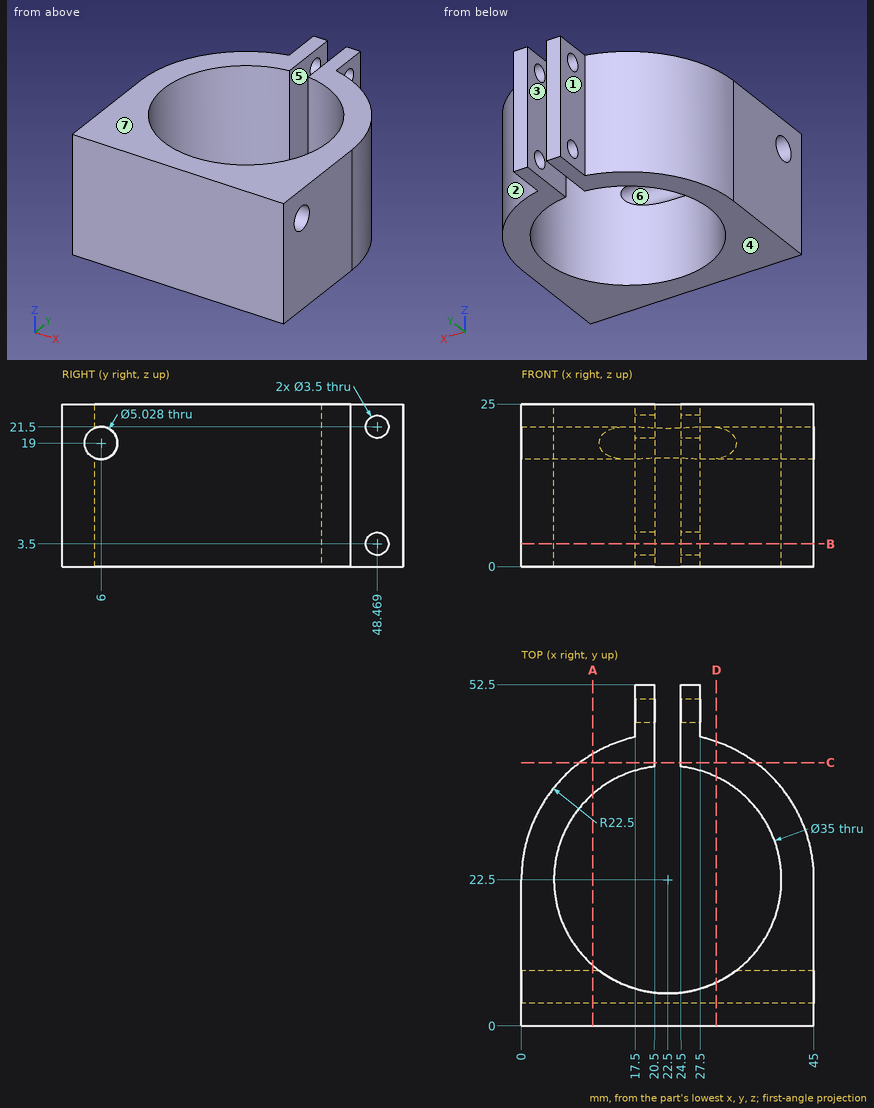
Design review of the part shown in the three views and the two pictorial views. Dimensions are in mm from the part's minimum x, y and z. A direction names the side the tool comes from. Coordinates: 2 decimals unless noted, no trailing zeros. Write each loop counter-clockwise with the first axis right and the second up, starting at its lowest first coordinate (ties: lowest second). Pieces come first, ordered by that corner, then holes.
(1) For pin 1 Ø3 at (y, z) = (48.47, 3.5) entering from -X; pin 2 Ø2 at (x, z) = (40.5, 16.5) entering from +Y; pin 3 Ø4 at (y, z) = (49, 7) entering from -X; pin 4 Ø10 at (y, z) = (36, 15) entering from -X, all flat-tipped, find the tip position at first contact; note any pin that passes through.
(2) Tool access review of the marked faces 1, 2 and 3: name each direction out of +Z, -Z, +X, -X, +Y, -Y from which nothing blocks a thin tool from reaching the whole face with its end or side.
(3) Add section B-B on z = 3.5. Give the boundary of the cut face in (x, y) (1 decimal), then the cut area to 3 significant figures.
(4) The part is to be moulded in two halves that separate along Z. For the marked faces 4, 5, 6 and 7, say which applies: +Z half, -Z half, draft (parallel to the pull), parting line (faces both ways), or undercut.
(5) Wall thickness on probe 1 along X at (y, z) = (22.5, 9); probe 2 along Z at (x, y) = (25.5, 47); probe 3 along X at (y, z) = (44.5, 8.25): over which ranges is each line inside the solid? List them lowest first.
(6) Add section D-D on x = 30. Give the boundary of the cut face in (y, z).
(7) Add section C-C on y = 40.5. Give the boundary of the cut face in (x, z), then the cut area to 3 significant figures.
(8) Add section A-A on x = 11. Give the boundary of the cut face in (y, z).
Answer sheet:
1. pin 1: passes through
1. pin 2: stops at y = 37.24
1. pin 3: stops at x = 17.5
1. pin 4: stops at x = 1.67
2. face 1: +Z, -Z, -X, +Y
2. face 2: +Z, -Z, +X, +Y
2. face 3: +Z, -Z, +Y
3. outline: (0, 0) - (45, 0) - (45, 22.5) arc R22.5 ccw to (27.5, 44.4) - (27.5, 46.7) - (24.5, 46.7) - (24.5, 39.9) arc R17.5 cw (long way) to (20.5, 39.9) - (20.5, 46.7) - (17.5, 46.7) - (17.5, 44.4) arc R22.5 ccw to (0, 22.5) - close; (17.5, 50.2) - (20.5, 50.2) - (20.5, 52.5) - (17.5, 52.5) - close; (24.5, 50.2) - (27.5, 50.2) - (27.5, 52.5) - (24.5, 52.5) - close
3. area: 851 mm2
4. face 4: -Z half
4. face 5: draft
4. face 6: undercut
4. face 7: +Z half
5. probe 1: x = 0 to 5, 40 to 45
5. probe 2: z = 0 to 2.55, 4.45 to 20.55, 22.45 to 25
5. probe 3: x = 17.5 to 20.5, 24.5 to 27.5
6. outline: (0, 0) - (6.69, 0) - (6.69, 16.58) arc R2.51 cw (long way) to (6.69, 21.42) - (6.69, 25) - (0, 25) - close; (38.31, 0) - (43.71, 0) - (43.71, 25) - (38.31, 25) - close
7. outline: (9, 0) - (20.5, 0) - (20.5, 25) - (9, 25) - close; (24.5, 0) - (36, 0) - (36, 25) - (24.5, 25) - close
7. area: 575 mm2
8. outline: (0, 0) - (9.31, 0) - (9.31, 25) - (0, 25) - close; (35.69, 0) - (41.84, 0) - (41.84, 25) - (35.69, 25) - close; hole circle Ø5.03 at (6, 19)
